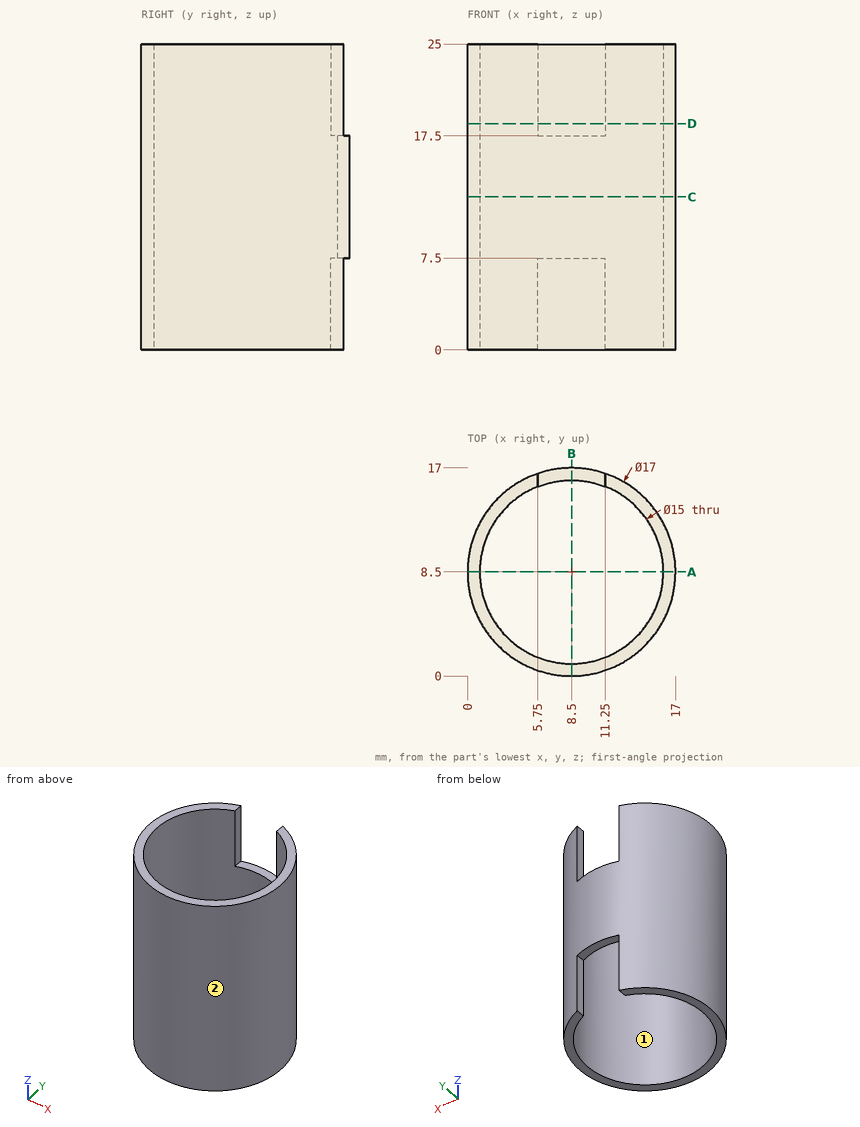
Here's the drawing with two shaded views (mm, measured from the low corner). I have some questions. Round coordinates to 2 decimals unless told otherwise and drop trailing zeros. Loops run counter-clockwise (first coordinate to the right, second up) from the corner with the lowest first, then second, coordinate; pieces in that order, holes last. Notation, with made-up numbers: M -15.75,76 L 39.25,76 A10 ccw 39.25,86 Z; hole C -13,5.5 d3. An arc over 180 degrees is marked long. Put each result on its own line as item: value.
Q1. Imagine slicing it at A-A (y = 8.5). Write out the boundary of the cut face in (x, z).
Check result:
outline: M 0,0 L 1,0 L 1,25 L 0,25 Z; M 16,0 L 17,0 L 17,25 L 16,25 Z
Q2. Imagine slicing it at C-C (z = 12.5). Write out the boundary of the cut face in (x, y), then the cut area to 3 significant figures.
Check result:
outline: C 8.5,8.5 d17; hole C 8.5,8.5 d15
area: 50.3 mm2
Q3. Imagine slicing it at B-B (x = 8.5). Write out the boundary of the cut face in (y, z).
Check result:
outline: M 0,0 L 1,0 L 1,25 L 0,25 Z; M 16,7.5 L 17,7.5 L 17,17.5 L 16,17.5 Z
Q4. Thinking about a two-plate mould opening in Y: for the marked faces 1 and 2, which applies, released by +Y, released by -Y, zero draft, split by the parting line, or undercut?
Check result:
face 1: undercut
face 2: split by the parting line
Q5. I need wall thicknesses on probe 1 along X at (y, z) = (8.5, 7); probe 2 along X at (y, z) = (6.75, 21.5); probe 3 along Y at (x, z) = (10.5, 16). Which ranges of each line are inside material? Lowest first, please.
Check result:
probe 1: 0 to 1, 16 to 17
probe 2: 0.18 to 1.21, 15.79 to 16.82
probe 3: 0.24 to 1.27, 15.73 to 16.76
Q6. Imagine slicing it at D-D (z = 18.5). Write out the boundary of the cut face in (x, y), then the cut area to 3 significant figures.
Check result:
outline: M 5.75,15.48 L 5.75,16.54 A8.5 ccw long 11.25,16.54 L 11.25,15.48 A7.5 cw long Z
area: 44.7 mm2
Q7. For pin 1 (5 mm diameter, centred on x = 6, y = 8.5, fed in from +Z); pin 2 (3 mm diameter, centred on y = 3.5, z = 13.5, fed in from +X); pin 3 (1.2 mm diameter, centred on y = 16, z = 21.5, fed in from -X); pin 4 (0.8 mm diameter, centred on x = 8, y = 16.5, fed in from -Z), each with a flat end and sliding along its axis, tell me the tip position at first contact or that it passes through.
Check result:
pin 1: through
pin 2: x = 16.25
pin 3: x = 3.54
pin 4: z = 7.5
